from build123d import *

# Parameters (mm, degrees)
SKETCH_1_W      = 22.5
SKETCH_1_H      = 12.5
EXTRUDE_1_DEPTH = 2
SKETCH_2_R      = 4
EXTRUDE_2_DEPTH = 1
SKETCH_3_R      = 3
EXTRUDE_3_DEPTH = 3.5
FILLET_1_R      = 0.5
FILLET_2_R      = 0.25


with BuildPart() as part:
    # 草图1 → 凸台-拉伸1 (new body)
    with BuildSketch(Plane(origin=(0, 0, 0), x_dir=(1, 0, 0), z_dir=(0, 1, 0))):
        with Locations((11.25, 6.25)):
            Rectangle(SKETCH_1_W, SKETCH_1_H)
    extrude(amount=EXTRUDE_1_DEPTH)

    # 草图2 → 凸台-拉伸2 (add)
    with BuildSketch(Plane(origin=(0, 2, 0), x_dir=(1, 0, 0), z_dir=(0, 1, 0))):
        with Locations(Location((6, 6.25, 0), (0, 0, 90))):
            Circle(SKETCH_2_R)
    extrude(amount=EXTRUDE_2_DEPTH)

    # 草图3 → 凸台-拉伸3 (add)
    with BuildSketch(Plane(origin=(0, 3, 0), x_dir=(1, 0, 0), z_dir=(0, 1, 0))):
        with Locations(Location((6, 6.25, 0), (0, 0, 270))):
            Circle(SKETCH_3_R)
    extrude(amount=EXTRUDE_3_DEPTH)

    # 圆角1
    fillet_1_edges = [part.edges().sort_by_distance(p)[0] for p in [
        (22.5, 2, -6.25),
        (6, 2, -2.25),
        (11.25, 2, -12.5),
        (0, 2, -6.25),
        (11.25, 0, -12.5),
        (22.5, 0, -6.25),
        (11.25, 0, 0),
        (0, 0, -6.25),
        (0, 1, -12.5),
        (22.5, 1, -12.5),
        (22.5, 1, 0),
        (0, 1, 0),
        (11.25, 2, 0),
    ]]
    fillet(fillet_1_edges, radius=FILLET_1_R)

    # 圆角2
    fillet_2_edges = [part.edges().sort_by_distance(p)[0] for p in [
        (6, 3, -2.25),
        (6, 6.5, -9.25),
    ]]
    fillet(fillet_2_edges, radius=FILLET_2_R)


solid = part.part
Input: part model. Units: mm. Frame: model coordinates. A direction names the side the tool comes from. Round coordinates to 2 decimals unless told otherwise and drop trailing zeros. Loops run counter-clockwise (first coordinate to the right, second up) from the corner with the lowest first, then second, coordinate; pieces in that order, holes last. Notation, with made-up numbers: (-27.75, 22) -> (-4.75, 22) arc R24 ccw to (-4.75, 33) -> close; hole circle Ø10 at (81, -23). An arc over 180 degrees is marked (long way). Answer as a JSON object with one key per item and string values. Group by question number.
1) Section query D-D on x = 6. Output: boundary loops of the cut face in (y, z), plus the area to 3 significant figures.
2) Section query C-C on y = 3.5. Output: boundary loops of the cut face in (x, z), plus the area to 3 significant figures.
3) Ray query, L1, parallel to Y at x = 15.5, z = -10.5; L2, parallel to Z at x = 5, y = 4.75; L3, parallel to Y at x = 7, z = -10. Return the intervals inside material, ascending.
4) Reachability of faces 1 (the cylindrical face through (3.338, 4.602, -4.866)), 2 (the flat face through (11, 0, -6)) from +Z, -Z, +X, -X, +Y, -Y: full face, straight path, thin tool, end or side. Return the list, or none.
5) Section query A-A on x = 16.5. Output: boundary loops of the cut face in (y, z).
6) Section query B-B on z = -6.25. Output: boundary loops of the cut face in (x, y), plus the area to 3 significant figures.
Reply:
{
 "1": {"outline": "(0, -12) arc R0.5 ccw to (0.5, -12.5) -> (1.5, -12.5) arc R0.5 ccw to (2, -12) -> (2, -10.75) arc R0.5 cw to (2.5, -10.25) -> (2.75, -10.25) arc R0.25 ccw to (3, -10) -> (3, -9.25) -> (6.25, -9.25) arc R0.25 ccw to (6.5, -9) -> (6.5, -3.5) arc R0.25 ccw to (6.25, -3.25) -> (3, -3.25) -> (3, -2.5) arc R0.25 ccw to (2.75, -2.25) -> (2.5, -2.25) arc R0.5 cw to (2, -1.75) -> (2, -0.5) arc R0.5 ccw to (1.5, 0) -> (0.5, 0) arc R0.5 ccw to (0, -0.5) -> close", "area": "53.8 mm2"},
 "2": {"outline": "circle Ø6 at (6, -6.25)", "area": "28.3 mm2"},
 "3": {"L1": "y = 0 to 2", "L2": "z = -9.08 to -3.42", "L3": "y = 0 to 2.96"},
 "4": {"face 1": "+Y", "face 2": "+Z, -Z, +X, -X, -Y"},
 "5": {"outline": "(0, -12) arc R0.5 ccw to (0.5, -12.5) -> (1.5, -12.5) arc R0.5 ccw to (2, -12) -> (2, -0.5) arc R0.5 ccw to (1.5, 0) -> (0.5, 0) arc R0.5 ccw to (0, -0.5) -> close"},
 "6": {"outline": "(0, 0.5) arc R0.5 ccw to (0.5, 0) -> (22, 0) arc R0.5 ccw to (22.5, 0.5) -> (22.5, 1.5) arc R0.5 ccw to (22, 2) -> (10.5, 2) arc R0.5 cw to (10, 2.5) -> (10, 2.75) arc R0.25 ccw to (9.75, 3) -> (9, 3) -> (9, 6.25) arc R0.25 ccw to (8.75, 6.5) -> (3.25, 6.5) arc R0.25 ccw to (3, 6.25) -> (3, 3) -> (2.25, 3) arc R0.25 ccw to (2, 2.75) -> (2, 2.5) arc R0.5 cw to (1.5, 2) -> (0.5, 2) arc R0.5 ccw to (0, 1.5) -> close", "area": "73.8 mm2"}
}
